from build123d import *

# Parameters (mm, degrees)
SKETCH2_W                                 = 188
SKETCH2_H                                 = 188
BOSS_EXTRUDE1_DEPTH                       = 30
FILLET1_R                                 = 19
CUT_EXTRUDE6_DEPTH                        = 4
CUT_EXTRUDE8_SVUOTAMENTO_DEPTH            = 26
CUT_EXTRUDE9_ALLOGGIAMENTO_FINESTRA_DEPTH = 3
BOSS_EXTRUDE2_DEPTH                       = 10
FILLET4_R                                 = 4
F_4_0MM_DOWEL_HOLE2_D                     = 4
CUT_EXTRUDE10_DEPTH                       = 6.6
CUT_EXTRUDE4_REACH                        = 217.044
SKETCH11_R                                = 1.5
CUT_EXTRUDE5_REACH                        = 217.044
SKETCH15_R                                = 1
CHAMFER1_SIZE                             = 4
CHAMFER1_SIZE_2                           = 3


with BuildPart() as part:
    # Sketch2 → Boss-Extrude1 (new body)
    with BuildSketch(Plane.XY):
        with Locations((-6, 6)):
            Rectangle(SKETCH2_W, SKETCH2_H)
    extrude(amount=BOSS_EXTRUDE1_DEPTH)

    # Fillet1
    fillet1_edges = [part.edges().sort_by_distance(p)[0] for p in [
        (88, -88, 15),
        (-100, -88, 15),
        (-100, 100, 15),
        (88, 100, 15),
    ]]
    fillet(fillet1_edges, radius=FILLET1_R)

    # Sketch18 → Cut-Extrude6 (cut)
    with BuildSketch(Plane.XY.offset(30)):
        with BuildLine():
            Line((-93.2, 81), (-93.2, -69))
            ThreePointArc((-93.2, -69), (-89.62670273, -77.62670273), (-81, -81.2))
            Line((-81, -81.2), (69, -81.2))
            ThreePointArc((69, -81.2), (77.62670273, -77.62670273), (81.2, -69))
            Line((81.2, -69), (81.2, 81))
            ThreePointArc((81.2, 81), (77.62670273, 89.62670273), (69, 93.2))
            Line((69, 93.2), (-81, 93.2))
            ThreePointArc((-81, 93.2), (-89.62670273, 89.62670273), (-93.2, 81))
        make_face()
    extrude(amount=-CUT_EXTRUDE6_DEPTH, mode=Mode.SUBTRACT)

    # Sketch19 → Cut-Extrude8-svuotamento (cut)
    with BuildSketch(Plane(origin=(0, 0, 0), x_dir=(-1, 0, 0), z_dir=(0, 0, -1))):
        with BuildLine():
            Line((-69, -84), (81, -84))
            ThreePointArc((81, -84), (91.606601718, -79.606601718), (96, -69))
            Line((96, -69), (96, 81))
            ThreePointArc((96, 81), (91.606601718, 91.606601718), (81, 96))
            Line((81, 96), (-69, 96))
            ThreePointArc((-69, 96), (-79.606601718, 91.606601718), (-84, 81))
            Line((-84, 81), (-84, -69))
            ThreePointArc((-84, -69), (-79.606601718, -79.606601718), (-69, -84))
        make_face()
    extrude(amount=-CUT_EXTRUDE8_SVUOTAMENTO_DEPTH, mode=Mode.SUBTRACT)

    # Sketch20 → Cut-Extrude9-alloggiamento-finestra (cut)
    with BuildSketch(Plane.XY.offset(30)):
        with BuildLine():
            Line((-94, 81), (-94, -69))
            ThreePointArc((-94, -69), (-90.192388155, -78.192388155), (-81, -82))
            Line((-81, -82), (69, -82))
            ThreePointArc((69, -82), (78.192388155, -78.192388155), (82, -69))
            Line((82, -69), (82, 81))
            ThreePointArc((82, 81), (78.192388155, 90.192388155), (69, 94))
            Line((69, 94), (-81, 94))
            ThreePointArc((-81, 94), (-90.192388155, 90.192388155), (-94, 81))
        make_face()
    extrude(amount=-CUT_EXTRUDE9_ALLOGGIAMENTO_FINESTRA_DEPTH, mode=Mode.SUBTRACT)

    # Sketch22 → Boss-Extrude2 (add)
    with BuildSketch(Plane(origin=(0, 0, 0), x_dir=(-1, 0, 0), z_dir=(0, 0, -1))):
        with BuildLine():
            Line((-84, 78), (-66, 78))
            Line((-66, 78), (-66, 96))
            Line((-66, 96), (-69, 96))
            ThreePointArc((-69, 96), (-79.606601718, 91.606601718), (-84, 81))
            Line((-84, 81), (-84, 78))
        make_face()
        with BuildLine():
            Line((81, 96), (78, 96))
            Line((78, 96), (78, 78))
            Line((78, 78), (96, 78))
            Line((96, 78), (96, 81))
            ThreePointArc((96, 81), (91.606601718, 91.606601718), (81, 96))
        make_face()
        with BuildLine():
            Line((78, -66), (78, -84))
            Line((78, -84), (81, -84))
            ThreePointArc((81, -84), (91.606601718, -79.606601718), (96, -69))
            Line((96, -69), (96, -66))
            Line((96, -66), (78, -66))
        make_face()
        with BuildLine():
            Line((-66, -66), (-84, -66))
            Line((-84, -66), (-84, -69))
            ThreePointArc((-84, -69), (-79.606601718, -79.606601718), (-69, -84))
            Line((-69, -84), (-66, -84))
            Line((-66, -84), (-66, -66))
        make_face()
    extrude(amount=-BOSS_EXTRUDE2_DEPTH)

    # Fillet4
    fillet4_edges = [part.edges().sort_by_distance(p)[0] for p in [
        (66, 78, 5),
        (-78, 78, 5),
        (-78, -66, 5),
        (66, -66, 5),
    ]]
    fillet(fillet4_edges, radius=FILLET4_R)

    # Ø4.0mm Dowel Hole2 (through all)
    with Locations(Plane(origin=(0, 0, 0), x_dir=(-1, 0, 0), z_dir=(0, 0, -1))):
        with Locations((-73, 85), (85, 85), (85, -73), (-73, -73)):
            Hole(F_4_0MM_DOWEL_HOLE2_D / 2)

    # Sketch30 → Cut-Extrude10 (cut)
    with BuildSketch(Plane(origin=(0, 0, 0), x_dir=(-1, 0, 0), z_dir=(0, 0, -1))):
        with BuildLine():
            Line((-69, -84), (81, -84))
            ThreePointArc((81, -84), (91.606601718, -79.606601718), (96, -69))
            Line((96, -69), (96, 81))
            ThreePointArc((96, 81), (91.606601718, 91.606601718), (81, 96))
            Line((81, 96), (-69, 96))
            ThreePointArc((-69, 96), (-79.606601718, 91.606601718), (-84, 81))
            Line((-84, 81), (-84, -69))
            ThreePointArc((-84, -69), (-79.606601718, -79.606601718), (-69, -84))
        make_face()
    extrude(amount=-CUT_EXTRUDE10_DEPTH, mode=Mode.SUBTRACT)

    # Sketch11 → Cut-Extrude4 (cut, up to next)
    with BuildSketch(Plane(origin=(0, 100, 0), x_dir=(1, 0, 0), z_dir=(0, 1, 0)), mode=Mode.PRIVATE) as cut_extrude4_sk1:
        with Locations(Location((-68.95500318, -14.324851484, 0), (0, 0, 270))):
            Circle(SKETCH11_R)
    cut_extrude4_tool1 = extrude(cut_extrude4_sk1.sketch, amount=-CUT_EXTRUDE4_REACH, mode=Mode.PRIVATE) & part.part
    add(cut_extrude4_tool1.solids().sort_by_distance((-68.955003, 100, 14.324851))[0], mode=Mode.SUBTRACT)

    # Sketch15 → Cut-Extrude5 (cut, up to next)
    with BuildSketch(Plane(origin=(-100, 0, 0), x_dir=(0, 0, -1), z_dir=(1, 0, 0)), mode=Mode.PRIVATE) as cut_extrude5_sk1:
        with Locations(Location((-9.460245724, -46.22788492, 0), (0, 0, 180))):
            Circle(SKETCH15_R)
    cut_extrude5_tool1 = extrude(cut_extrude5_sk1.sketch, amount=CUT_EXTRUDE5_REACH, mode=Mode.PRIVATE) & part.part
    # Sketch15 → Cut-Extrude5 (cut, up to next)
    with BuildSketch(Plane(origin=(-100, 0, 0), x_dir=(0, 0, -1), z_dir=(1, 0, 0)), mode=Mode.PRIVATE) as cut_extrude5_sk2:
        with BuildLine():
            Line((-8.900245724, -53.495303579), (-9.460245724, -53.495303579))
            ThreePointArc((-9.460245724, -53.495303579), (-10.73303793, -54.022511373), (-11.260245724, -55.295303579))
            Line((-11.260245724, -55.295303579), (-11.260245724, -61.645303576))
            ThreePointArc((-11.260245724, -61.645303576), (-10.73303793, -62.918095782), (-9.460245724, -63.445303576))
            Line((-9.460245724, -63.445303576), (-8.900245724, -63.445303576))
            ThreePointArc((-8.900245724, -63.445303576), (-7.627453518, -62.918095782), (-7.100245724, -61.645303576))
            Line((-7.100245724, -61.645303576), (-7.100245724, -55.295303579))
            ThreePointArc((-7.100245724, -55.295303579), (-7.627453518, -54.022511373), (-8.900245724, -53.495303579))
        make_face()
    cut_extrude5_tool2 = extrude(cut_extrude5_sk2.sketch, amount=CUT_EXTRUDE5_REACH, mode=Mode.PRIVATE) & part.part
    add(cut_extrude5_tool1.solids().sort_by_distance((-100, -46.227885, 9.460246))[0], mode=Mode.SUBTRACT)
    add(cut_extrude5_tool2.solids().sort_by_distance((-100, -58.470304, 9.180246))[0], mode=Mode.SUBTRACT)

    # Chamfer1
    # the kernel refuses this chamfer: 4, 3 mm, written as the material it adds along each edge
    with BuildSketch(Plane(origin=(69, -84, 26), x_dir=(0, -0.023249527748764737, -0.9997296931968459), z_dir=(-1, 0, 0))) as chamfer1_piece_1_section:
        Polygon((CHAMFER1_SIZE * 0.999729693197, -CHAMFER1_SIZE * 0.0232495277488), (-CHAMFER1_SIZE_2 * 0.0232495277488, -CHAMFER1_SIZE_2 * 0.999729693197), (0, 0), align=None)
    chamfer1_piece_1 = extrude(amount=150, mode=Mode.PRIVATE)
    chamfer1_piece_1 = split(chamfer1_piece_1, bisect_by=Plane(origin=(-6, -81.2, 24.654371932), z_dir=(0, -1, 0)), keep=Keep.TOP, mode=Mode.PRIVATE)
    add(chamfer1_piece_1)
    with BuildSketch(Plane(origin=(-81, -69, 26), x_dir=(0, -1, 0), z_dir=(1, 0, 0))) as chamfer1_piece_2_section:
        Polygon((15 - CHAMFER1_SIZE_2, 0), (15, CHAMFER1_SIZE), (15, 0), align=None)
    chamfer1_piece_2 = revolve(axis=Axis((-81, -69, 26), (0, 0, -1)), revolution_arc=90, mode=Mode.PRIVATE)
    chamfer1_piece_2 = chamfer1_piece_2 - Plane(origin=(-81, -69, 24.826857266), x_dir=(-1, 0, 0), z_dir=(0, 0, 1)) * Cylinder(12.2, 60, mode=Mode.PRIVATE)
    add(chamfer1_piece_2)
    with BuildSketch(Plane(origin=(69, -69, 26), x_dir=(1, 0, 0), z_dir=(0, 1, 0))) as chamfer1_piece_3_section:
        Polygon((15 - CHAMFER1_SIZE_2, 0), (15, CHAMFER1_SIZE), (15, 0), align=None)
    chamfer1_piece_3 = revolve(axis=Axis((69, -69, 26), (0, 0, -1)), revolution_arc=90, mode=Mode.PRIVATE)
    chamfer1_piece_3 = chamfer1_piece_3 - Plane(origin=(69, -69, 24.826857266), x_dir=(0, -1, 0), z_dir=(0, 0, 1)) * Cylinder(12.2, 60, mode=Mode.PRIVATE)
    add(chamfer1_piece_3)
    with BuildSketch(Plane(origin=(-96, -69, 26), x_dir=(-0.023249527748764737, 0, -0.9997296931968459), z_dir=(0, 1, 0))) as chamfer1_piece_4_section:
        Polygon((CHAMFER1_SIZE * 0.999729693197, -CHAMFER1_SIZE * 0.0232495277488), (-CHAMFER1_SIZE_2 * 0.0232495277488, -CHAMFER1_SIZE_2 * 0.999729693197), (0, 0), align=None)
    chamfer1_piece_4 = extrude(amount=150, mode=Mode.PRIVATE)
    chamfer1_piece_4 = split(chamfer1_piece_4, bisect_by=Plane(origin=(-93.2, 6, 24.654371932), z_dir=(-1, 0, 0)), keep=Keep.TOP, mode=Mode.PRIVATE)
    add(chamfer1_piece_4)
    with BuildSketch(Plane(origin=(84, 81, 26), x_dir=(0.023249527748764737, 0, -0.9997296931968459), z_dir=(0, -1, 0))) as chamfer1_piece_5_section:
        Polygon((CHAMFER1_SIZE * 0.999729693197, -CHAMFER1_SIZE * 0.0232495277488), (-CHAMFER1_SIZE_2 * 0.0232495277488, -CHAMFER1_SIZE_2 * 0.999729693197), (0, 0), align=None)
    chamfer1_piece_5 = extrude(amount=150, mode=Mode.PRIVATE)
    chamfer1_piece_5 = split(chamfer1_piece_5, bisect_by=Plane(origin=(81.2, 6, 24.654371932), z_dir=(1, 0, 0)), keep=Keep.TOP, mode=Mode.PRIVATE)
    add(chamfer1_piece_5)
    with BuildSketch(Plane(origin=(-81, 81, 26), x_dir=(-1, 0, 0), z_dir=(0, -1, 0))) as chamfer1_piece_6_section:
        Polygon((15 - CHAMFER1_SIZE_2, 0), (15, CHAMFER1_SIZE), (15, 0), align=None)
    chamfer1_piece_6 = revolve(axis=Axis((-81, 81, 26), (0, 0, -1)), revolution_arc=90, mode=Mode.PRIVATE)
    chamfer1_piece_6 = chamfer1_piece_6 - Plane(origin=(-81, 81, 24.826857266), x_dir=(0, 1, 0), z_dir=(0, 0, 1)) * Cylinder(12.2, 61, mode=Mode.PRIVATE)
    add(chamfer1_piece_6)
    with BuildSketch(Plane(origin=(69, 81, 26), x_dir=(0, 1, 0), z_dir=(-1, 0, 0))) as chamfer1_piece_7_section:
        Polygon((15, CHAMFER1_SIZE), (15 - CHAMFER1_SIZE_2, 0), (15, 0), align=None)
    chamfer1_piece_7 = revolve(axis=Axis((69, 81, 26), (0, 0, -1)), revolution_arc=90, mode=Mode.PRIVATE)
    chamfer1_piece_7 = chamfer1_piece_7 - Plane(origin=(69, 81, 24.516674107), x_dir=(1, 0, 0), z_dir=(0, 0, 1)) * Cylinder(12.2, 61, mode=Mode.PRIVATE)
    add(chamfer1_piece_7)
    with BuildSketch(Plane(origin=(-81, 96, 26), x_dir=(0, 0.023249527748764737, -0.9997296931968459), z_dir=(1, 0, 0))) as chamfer1_piece_8_section:
        Polygon((CHAMFER1_SIZE * 0.999729693197, -CHAMFER1_SIZE * 0.0232495277488), (-CHAMFER1_SIZE_2 * 0.0232495277488, -CHAMFER1_SIZE_2 * 0.999729693197), (0, 0), align=None)
    chamfer1_piece_8 = extrude(amount=150, mode=Mode.PRIVATE)
    chamfer1_piece_8 = split(chamfer1_piece_8, bisect_by=Plane(origin=(-6, 93.2, 24.654371932), z_dir=(0, 1, 0)), keep=Keep.TOP, mode=Mode.PRIVATE)
    add(chamfer1_piece_8)


solid = part.part
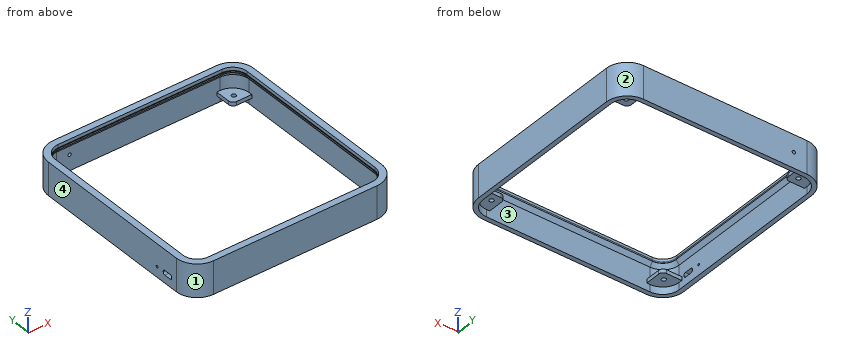
For this review, take the finished solid that the model builds, in its own axes (mm). Face numbers are marked on the shaded views. Round coordinates to 2 decimals unless told otherwise and drop trailing zeros. Write each loop counter-clockwise with the first axis right and the second up, starting at its lowest first coordinate (ties: lowest second). Pieces come first, ordered by that corner, then holes. Notation, with made-up numbers: (19.5, 67) - (54.5, 67) arc R8 cw to (54.5, 75) - close; hole circle Ø7 at (-1, 41.5). An arc over 180 degrees is marked (long way). Use a Markdown table: item, result.
Q1. We need section A-A (x = 39.5). Give the boundary of the cut face in (y, z), plus the area to 3 significant figures.
Derived:
| item | result |
|---|---|
| outline | (-88, 0) - (-84, 0) - (-84, 22) - (-81.2, 25.73) - (-81.2, 27) - (-82, 27) - (-82, 30) - (-88, 30) - close; (93.2, 25.73) - (96, 22) - (96, 0) - (100, 0) - (100, 30) - (94, 30) - (94, 27) - (93.2, 27) - close |
| area | 270 mm2 |
Q2. The part is to be moulded in two halves that separate along Y. For the marked faces 1, 2, 3 and 4, say which applies: pulls with the +Y half, pulls with the -Y half, needs draft (parallel to the pull), parting line crosses it, or undercut.
Derived:
| item | result |
|---|---|
| face 1 | pulls with the -Y half |
| face 2 | pulls with the +Y half |
| face 3 | undercut |
| face 4 | needs draft |
Q3. We need section B-B (y = -27). Give the boundary of the cut face in (x, z), plus the area to 3 significant figures.
Derived:
| item | result |
|---|---|
| outline | (-100, 0) - (-96, 0) - (-96, 22) - (-93.2, 25.73) - (-93.2, 27) - (-94, 27) - (-94, 30) - (-100, 30) - close; (81.2, 25.73) - (84, 22) - (84, 0) - (88, 0) - (88, 30) - (82, 30) - (82, 27) - (81.2, 27) - close |
| area | 270 mm2 |
Q4. Wall thickness on line 1 along X through (y, z) = (40.5, 4.5); line 2 along Y through (x, z) = (-85, 7.5); line 3 along Y through (x, z) = (-46, 11.75): over which ranges is each line inside the solid? List them lowest first.
Derived:
| item | result |
|---|---|
| line 1 | x = -100 to -96, 84 to 88 |
| line 2 | y = -87.57 to -75, -71 to -66, 78 to 83, 87 to 99.57 |
| line 3 | y = -88 to -84, 96 to 100 |
Q5. Clearance check with flat-ended pins moving along their axes: pin 1 (5.5 mm diameter, centred on x = -85, y = 86, fed in from -Z); pin 2 (2.5 mm diameter, centred on x = -68.96, z = 14.32, fed in from +Y); pin 3 (1.7 mm diameter, centred on x = -90.5, z = 9, fed in from +Y); pin 4 (14.5 mm diameter, centred on x = 78, y = -77, fed in from +Z). State where each tip first meets the part, or that it passes through.
Derived:
| item | result |
|---|---|
| pin 1 | stops at z = 6.6 |
| pin 2 | stops at y = -84 |
| pin 3 | stops at y = 97.92 |
| pin 4 | stops at z = 30 |
